```python
from build123d import *

# Parameters (mm, degrees)
F0_R     = 44.45
F0_R_2   = 38.1
F1_DEPTH = 25.4
F3_R     = 31.75
F4_DEPTH = 2.54


with BuildPart() as f1:
    # F0 (on Right) → F1 (new body)
    with BuildSketch(Plane.YZ):
        Circle(F0_R)
        Circle(F0_R_2, mode=Mode.SUBTRACT)
    extrude(amount=F1_DEPTH)

    # F3 (on offset) → F4 (join, symmetric)
    with BuildSketch(Plane.XY.offset(44.45)):
        with Locations((12.7, 0)):
            Circle(F3_R)
    extrude(amount=F4_DEPTH, both=True)


solid = f1.part
```
The model under review builds one solid part; all positions refer to its coordinate system, in mm. A direction names the side the tool comes from. Round coordinates to 2 decimals unless told otherwise and drop trailing zeros. Order: outer loops, then holes, each group sorted by start corner. A loop starts at its lowest first (then second) coordinate and runs counter-clockwise, first axis right, second up.
Item 1: For pin 1 (6 mm diameter, centred on x = 10, z = -28.5, fed in from -Y); pin 2 (12 mm diameter, centred on x = 19, y = -35, fed in from +Z); pin 3 (3 mm diameter, centred on x = 2.5, y = -34, fed in from +Z); pin 4 (1.5 mm diameter, centred on x = 6, y = -23, fed in from -Z), all flat-tipped, find the tip position at first contact; note any pin that passes through.
Working result:
pin 1: stops at y = -36.41
pin 2: stops at z = 46.99
pin 3: stops at z = 30.32
pin 4: stops at z = -38.48
Item 2: Add section D-D, the plane x = 17.5. State the section outline as (y, z) points, and give its area (3 significant figures).
Working result:
outline: (-31.39, 41.91) - (-14.81, 41.91) arc R44.45 ccw (long way) to (14.81, 41.91) - (31.39, 41.91) - (31.39, 46.99) - (-31.39, 46.99) - close; hole circle Ø76.2 at (0, 0)
area: 1,920 mm2
Item 3: Draft analysis for pull direction Z (two halves, no side actions). For faces 5 (the cylindrical face through (12.522, -1.743, -44.416)), 6 (the cylindrical face through (5.817, -30.995, 44.486)), 7 (the flat face through (12, 0, 46.99)), state which applies: released by +Z, released by -Z, zero draft, split by the parting line, or undercut.
Working result:
face 5: undercut
face 6: zero draft
face 7: released by +Z
Item 4: Machinability: for faces 1 (the flat face through (26, 0, 41.91)), 2 (the cylindrical face through (12.522, -30.235, -23.183)), 3 (the flat face through (0, 13, -36)), 4 (the flat face through (25.4, 13, -36)), which of the approach directions +Z, -Z, +X, -X, +Y, -Y give a long, thin tool a straight path to every point of the face, cutting with its end or side? Answer none if there is none.
Working result:
face 1: none
face 2: +X, -X
face 3: -Z, -X, +Y, -Y
face 4: -Z, +X, +Y, -Y
Item 5: Add section A-A, the plane y = 0. State the section outline as (x, z) points.
Working result:
outline: (-19.05, 41.91) - (0, 41.91) - (0, 38.1) - (25.4, 38.1) - (25.4, 41.91) - (44.45, 41.91) - (44.45, 46.99) - (-19.05, 46.99) - close; (0, -44.45) - (25.4, -44.45) - (25.4, -38.1) - (0, -38.1) - close
Item 6: Add section B-B, the plane z = -3. State the section outline as (x, y) points.
Working result:
outline: (0, -44.35) - (25.4, -44.35) - (25.4, -37.98) - (0, -37.98) - close; (0, 37.98) - (25.4, 37.98) - (25.4, 44.35) - (0, 44.35) - close
Item 7: To check wall thickness, follow probe 1 along Z at (x, y) = (20, 0); probe 2 along Z at (x, y) = (12, -18); probe 3 along Z at (x, y) = (-16, 13.5). State the ranges of each line that lie inside material, in increasing order.
Working result:
probe 1: z = -44.45 to -38.1, 38.1 to 46.99
probe 2: z = -40.64 to -33.58, 33.58 to 40.64, 41.91 to 46.99
probe 3: z = 41.91 to 46.99
Item 8: Add section C-C, the plane y = 18.5. State the section outline as (x, z) points, and give its area (3 significant figures).
Working result:
outline: (-13.1, 41.91) - (38.5, 41.91) - (38.5, 46.99) - (-13.1, 46.99) - close; (0, -40.42) - (25.4, -40.42) - (25.4, -33.31) - (0, -33.31) - close; (0, 33.31) - (25.4, 33.31) - (25.4, 40.42) - (0, 40.42) - close
area: 623 mm2
